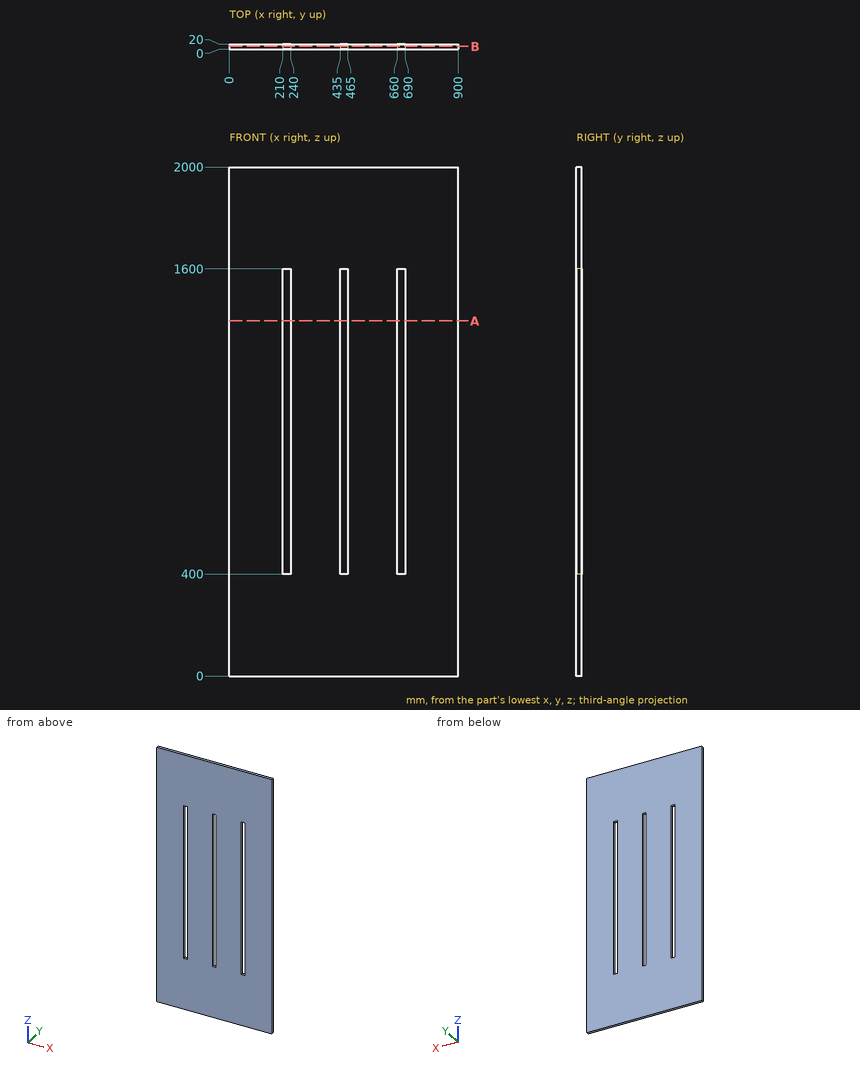
Design review of the part shown in the three views and the two pictorial views. Dimensions are in mm from the part's minimum x, y and z. Round coordinates to 2 decimals unless told otherwise and drop trailing zeros. Order: outer loops, then holes, each group sorted by start corner. A loop starts at its lowest first (then second) coordinate and runs counter-clockwise, first axis right, second up. Notation, with made-up numbers: (20, 45) -> (58, 45) arc R22 ccw to (58, 64) -> close; hole circle Ø5 at (20.5, 42). An arc over 180 degrees is marked (long way). Write item = value, one per line. Start each with the question number.
1) Take a section at B-B on y = 10.25. State the section outline as (x, z) points.
2) Take a section at A-A on z = 1396. State the section outline as (x, y) points, plus the area to 3 significant figures.
3) Insertion check: pin 1 (10 mm diameter, centred on x = 459.5, z = 878, fed in from -Y). The pin has a flat end and moves straight along its axis. Give the tip position at first contact, or say it passes through.
4) To check wall thickness, follow line 1 (X direction, y = 13.25, z = 1449.5); line 2 (Z direction, x = 213.5, y = 18). State the ranges of each line that lie inside material, in increasing order. Write a range as from..to.
Verdict:
q1.outline = (0, 0) -> (900, 0) -> (900, 2000) -> (0, 2000) -> close; hole (210, 400) -> (240, 400) -> (240, 1600) -> (210, 1600) -> close; hole (435, 400) -> (465, 400) -> (465, 1600) -> (435, 1600) -> close; hole (660, 400) -> (690, 400) -> (690, 1600) -> (660, 1600) -> close
q2.outline = (0, 0) -> (210, 0) -> (210, 20) -> (0, 20) -> close; (240, 0) -> (435, 0) -> (435, 20) -> (240, 20) -> close; (465, 0) -> (660, 0) -> (660, 20) -> (465, 20) -> close; (690, 0) -> (900, 0) -> (900, 20) -> (690, 20) -> close
q2.area = 16,200 mm2
q3.pin_1 = through
q4.line_1 = 0..210, 240..435, 465..660, 690..900
q4.line_2 = 0..400, 1600..2000
